Part print with two shaded views. Sizes in mm from the minimum x, y, z corner. A direction names the side the tool comes from. Give positions to 0.01 mm unless a question says otherwise; leave off trailing zeros. Order: outer loops, then holes, each group sorted by start corner. A loop starts at its lowest first (then second) coordinate and runs counter-clockwise, first axis right, second up. Notation, with made-up numbers: M -8.5,-24 L 41.5,-24 A16 cw 41.5,6 Z; hole C 9.25,-39 d1. An arc over 180 degrees is marked long. Return JSON: item names as keys, results as strings. Group by question number.
1. Two-plate mould, pull along Z, no slides. Class the marked faces 1, 2 and 3: released by +Z, released by -Z, zero draft, split by the parting line, or undercut.
2. Slice it at C-C on z = 4. List the corners of the cut face in (x, y).
3. Wall check: probe 1 along Y at (x, z) = (10, 33.6); probe 2 along Z at (x, y) = (18.75, 10); probe 3 along Y at (x, z) = (9.5, 4). Give the ranges that are in metal, low to high. Write a range as [from, to].
4. Slice it at D-D on y = 3.5. List the corners of the cut face in (x, z).
5. Slice it at A-A on y = 10. List the corners of the cut face in (x, z).
6. Pin check, flat tips, straight feed: pin 1 (2.5 mm diameter, centred on x = 17, y = 10, fed in from -Z); pin 2 (1 mm diameter, centred on x = 14, z = 31, fed in from +Y); pin 3 (12 mm diameter, centred on y = 7, z = 15, fed in from +X); pin 4 (12 mm diameter, centred on y = 11, z = 11.5, fed in from -X). Stop position of each tip, or through.
7. 3-axis set-ups, long thin cutter, end or side, ignore diameter. For the marked faces 4 and 5: which of +Z, -Z, +X, -X, +Y, -Y reach the whole face in a straight line?
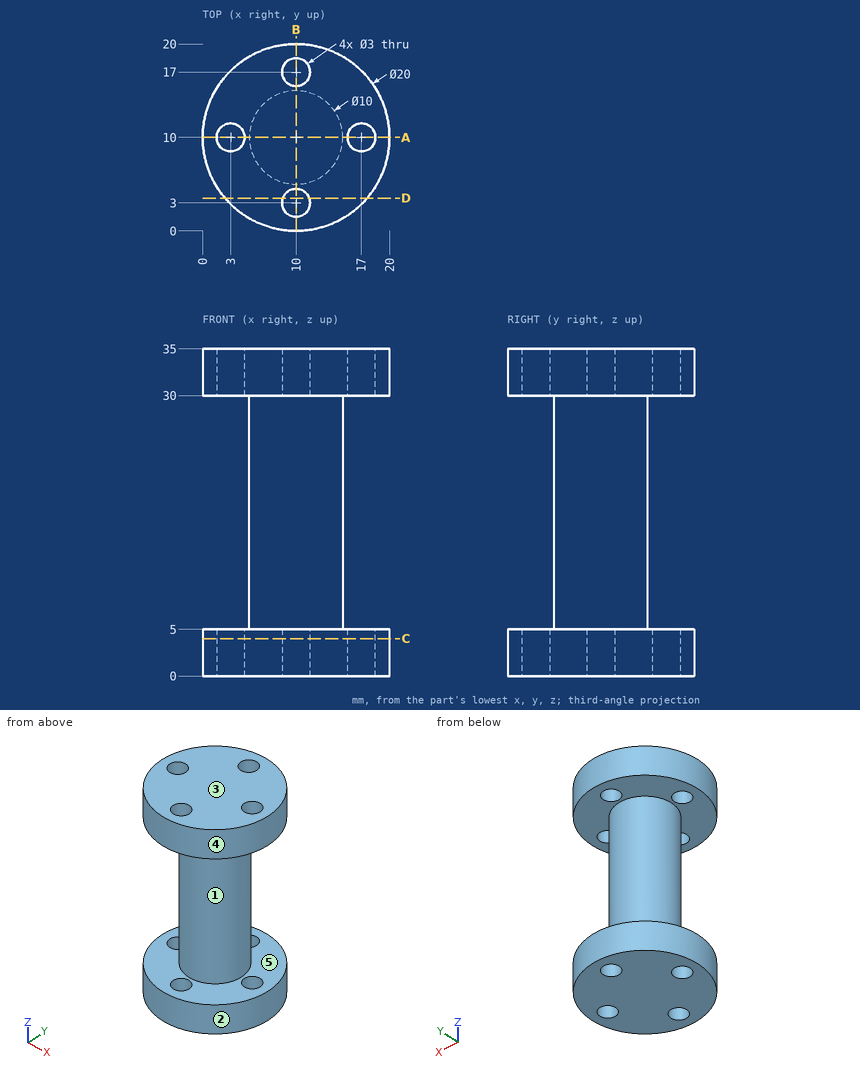
Result:
{
 "1": {"face 1": "undercut", "face 2": "zero draft", "face 3": "released by +Z"},
 "2": {"outline": "C 10,10 d20; hole C 3,10 d3; hole C 10,3 d3; hole C 10,17 d3; hole C 17,10 d3"},
 "3": {"probe 1": "y = [0, 1.5], [4.5, 15.5], [18.5, 20]", "probe 2": "z = [0, 5], [30, 35]", "probe 3": "y = [0.01, 1.59], [4.41, 15.59], [18.41, 19.99]"},
 "4": {"outline": "M 2.4,0 L 8.59,0 L 8.59,5 L 2.4,5 Z; M 2.4,30 L 8.59,30 L 8.59,35 L 2.4,35 Z; M 11.41,0 L 17.6,0 L 17.6,5 L 11.41,5 Z; M 11.41,30 L 17.6,30 L 17.6,35 L 11.41,35 Z"},
 "5": {"outline": "M 0,0 L 1.5,0 L 1.5,5 L 0,5 Z; M 0,30 L 1.5,30 L 1.5,35 L 0,35 Z; M 4.5,0 L 15.5,0 L 15.5,5 L 15,5 L 15,30 L 15.5,30 L 15.5,35 L 4.5,35 L 4.5,30 L 5,30 L 5,5 L 4.5,5 Z; M 18.5,0 L 20,0 L 20,5 L 18.5,5 Z; M 18.5,30 L 20,30 L 20,35 L 18.5,35 Z"},
 "6": {"pin 1": "passes through", "pin 2": "stops at y = 19.37", "pin 3": "stops at x = 15", "pin 4": "stops at x = 5"},
 "7": {"face 4": "+Z, -Z", "face 5": "none"}
}
